```python
from build123d import *

# Parameters (mm, degrees)
SKETCH1_W           = 100
SKETCH1_H           = 100
SKETCH1_R           = 6
BOSS_EXTRUDE1_DEPTH = 4
SKETCH1_3_W         = 4
SKETCH1_3_H         = 99
SKETCH1_3_W_2       = 99
SKETCH1_3_H_2       = 4
BOSS_EXTRUDE3_DEPTH = 34
FILLET3_R           = 2
SKETCH2_R           = 2
SKETCH2_R_2         = 1.75
CUT_EXTRUDE1_DEPTH  = 4
SKETCH3_R           = 2
SKETCH3_R_2         = 1.75
CUT_EXTRUDE2_DEPTH  = 4
SKETCH4_R           = 2
SKETCH4_R_2         = 1.75
CUT_EXTRUDE3_DEPTH  = 4
SKETCH5_R           = 2
SKETCH5_R_2         = 1.75
CUT_EXTRUDE4_DEPTH  = 4


with BuildPart() as part:
    # Sketch1 → Boss-Extrude1 (new body)
    with BuildSketch(Plane.XY):
        with Locations((-48.16802168, -14.386178862)):
            Rectangle(SKETCH1_W, SKETCH1_H)
        with Locations((-88.16802168, -54.386178862)):
            Circle(SKETCH1_R, mode=Mode.SUBTRACT)
        with Locations((-8.16802168, -54.386178862)):
            Circle(SKETCH1_R, mode=Mode.SUBTRACT)
        with Locations((-8.16802168, 25.613821138)):
            Circle(SKETCH1_R, mode=Mode.SUBTRACT)
        with Locations((-88.16802168, 25.613821138)):
            Circle(SKETCH1_R, mode=Mode.SUBTRACT)
    extrude(amount=BOSS_EXTRUDE1_DEPTH)

    # Sketch1<3> → Boss-Extrude3 (add)
    with BuildSketch(Plane.XY):
        with Locations((-100.16802168, -14.386178862)):
            Rectangle(SKETCH1_3_W, SKETCH1_3_H)
        with Locations((-48.16802168, 37.613821138)):
            Rectangle(SKETCH1_3_W_2, SKETCH1_3_H_2)
        with Locations((3.83197832, -14.386178862)):
            Rectangle(SKETCH1_3_W, SKETCH1_3_H)
        with Locations((-48.16802168, -66.386178862)):
            Rectangle(SKETCH1_3_W_2, SKETCH1_3_H_2)
    extrude(amount=BOSS_EXTRUDE3_DEPTH)

    # Fillet3
    fillet3_edges = [part.edges().sort_by_distance(p)[0] for p in [
        (-102.16802168, -14.386178862, 0),
        (-48.16802168, 39.613821138, 0),
        (5.83197832, -14.386178862, 0),
        (-48.16802168, -68.386178862, 0),
    ]]
    fillet(fillet3_edges, radius=FILLET3_R)

    # Sketch2 → Cut-Extrude1 (cut)
    with BuildSketch(Plane.ZY.offset(102.16802168)):
        with Locations((25, 31.113821138)):
            Circle(SKETCH2_R)
        with Locations((25, -59.886178862)):
            Circle(SKETCH2_R)
        with Locations((11, 31.113821138)):
            Circle(SKETCH2_R)
        with Locations((11, -59.886178862)):
            Circle(SKETCH2_R)
        with Locations((11, 23.713821138)):
            Circle(SKETCH2_R_2)
        with Locations((11, -52.486178862)):
            Circle(SKETCH2_R_2)
    extrude(amount=-CUT_EXTRUDE1_DEPTH, mode=Mode.SUBTRACT)

    # Sketch3 → Cut-Extrude2 (cut)
    with BuildSketch(Plane.XZ.offset(68.386178862)):
        with Locations((-93.66802168, 25)):
            Circle(SKETCH3_R)
        with Locations((-2.66802168, 25)):
            Circle(SKETCH3_R)
        with Locations((-93.66802168, 11)):
            Circle(SKETCH3_R)
        with Locations((-2.66802168, 11)):
            Circle(SKETCH3_R)
        with Locations((-86.26802168, 11)):
            Circle(SKETCH3_R_2)
        with Locations((-9.56802168, 11)):
            Circle(SKETCH3_R_2)
    extrude(amount=-CUT_EXTRUDE2_DEPTH, mode=Mode.SUBTRACT)

    # Sketch4 → Cut-Extrude3 (cut)
    with BuildSketch(Plane(origin=(5.83197832, 0, 0), x_dir=(0, 0, -1), z_dir=(1, 0, 0))):
        with Locations((-25, -59.886178862)):
            Circle(SKETCH4_R)
        with Locations((-25, 31.113821138)):
            Circle(SKETCH4_R)
        with Locations((-11, -59.886178862)):
            Circle(SKETCH4_R)
        with Locations((-11, 31.113821138)):
            Circle(SKETCH4_R)
        with Locations((-11, -52.486178862)):
            Circle(SKETCH4_R_2)
        with Locations((-11, 23.713821138)):
            Circle(SKETCH4_R_2)
    extrude(amount=-CUT_EXTRUDE3_DEPTH, mode=Mode.SUBTRACT)

    # Sketch5 → Cut-Extrude4 (cut)
    with BuildSketch(Plane(origin=(0, 39.613821138, 0), x_dir=(1, 0, 0), z_dir=(0, 1, 0))):
        with Locations((-93.66802168, -25)):
            Circle(SKETCH5_R)
        with Locations((-2.66802168, -25)):
            Circle(SKETCH5_R)
        with Locations((-93.66802168, -11)):
            Circle(SKETCH5_R)
        with Locations((-2.66802168, -11)):
            Circle(SKETCH5_R)
        with Locations((-86.26802168, -11)):
            Circle(SKETCH5_R_2)
        with Locations((-10.06802168, -11)):
            Circle(SKETCH5_R_2)
    extrude(amount=-CUT_EXTRUDE4_DEPTH, mode=Mode.SUBTRACT)


solid = part.part
```
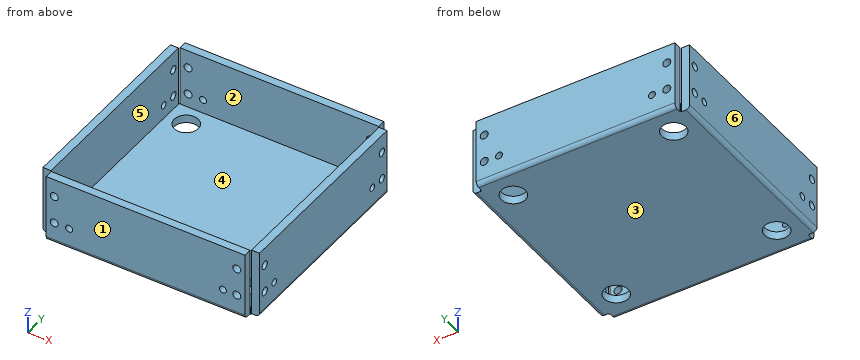
Read the model definition and answer for the solid it produces. Units are mm, in the model's axes. Face numbers are marked on the shaded views. A direction names the side the tool comes from. Round coordinates to 2 decimals unless told otherwise and drop trailing zeros. Write each loop counter-clockwise with the first axis right and the second up, starting at its lowest first coordinate (ties: lowest second). Pieces come first, ordered by that corner, then holes. Notation, with made-up numbers: (-9, -31.5) -> (49, -31.5) arc R33 cw to (49, 6.5) -> close; hole circle Ø10 at (51.5, -13.5). An arc over 180 degrees is marked (long way). Answer in a Markdown table with one row per item. Add a question column.
1) Find section C-C, the plane y = -6.5. Determine the outline of the cut face in (x, z).
2) Find section B-B, the plane x = -66.5. Determine the outline of the cut face in (y, z).
3) Find section D-D, the plane z = 25. State how many separate pieces and enclosed holes the cut face has, and give its area (3 significant figures).
4) Which of the six approach directions +Z, -Z, +X, -X, +Y, -Y give full straight-line access (tool end or side, diameter ignored) to the marked faces 1 and 2?
5) Given P1, Ø3, axis at y = -59.89, z = 11, coming from the -X side; P2, Ø4.5, axis at y = -66, z = 20, coming from the +X side, each flat-ended and moving along its own axis, determine where each tip first touches the part or whether it passes through.
6) Determine the mould class of the marked faces 3, 4, 5 and 6 for opening direction X: pulls with the +X half, pulls with the -X half, needs draft (parallel to the pull), parting line crosses it, or undercut.
7) Consider line 1 (Y direction, x = -100, z = 11); line 2 (Y direction, x = -31.5, z = 10.5); line 3 (X direction, y = -38.5, z = 19.5). Determine where each line is inside the solid, lowest interval first.
8) Find section A-A, the plane z = 6.5. Determine the outline of the cut face in (x, y).
Findings below:
| question | item | result |
|---|---|---|
| 1 | outline | (-102.17, 2) arc R2 ccw to (-100.17, 0) -> (3.83, 0) arc R2 ccw to (5.83, 2) -> (5.83, 34) -> (1.83, 34) -> (1.83, 4) -> (-98.17, 4) -> (-98.17, 34) -> (-102.17, 34) -> close |
| 2 | outline | (-68.39, 2) arc R2 ccw to (-66.39, 0) -> (37.61, 0) arc R2 ccw to (39.61, 2) -> (39.61, 34) -> (35.61, 34) -> (35.61, 4) -> (-64.39, 4) -> (-64.39, 34) -> (-68.39, 34) -> close |
| 3 | separate pieces | 12 |
| 3 | enclosed holes | 0 |
| 3 | area | 1,460 mm² |
| 4 | face 1 | +Z, -Z, +X, -X, -Y |
| 4 | face 2 | +Z, +X, -X |
| 5 | P1 | through |
| 5 | P2 | x = 5.83 |
| 6 | face 3 | needs draft |
| 6 | face 4 | undercut |
| 6 | face 5 | undercut |
| 6 | face 6 | pulls with the -X half |
| 7 | line 1 | -63.89 to -61.89, -57.89 to -54.24, -50.74 to 21.96, 25.46 to 29.11, 33.11 to 35.11 |
| 7 | line 2 | -68.39 to -64.39, 35.61 to 39.61 |
| 7 | line 3 | -102.17 to -98.17, 1.83 to 5.83 |
| 8 | outline | (-102.17, -63.89) -> (-98.17, -63.89) -> (-98.17, 35.11) -> (-102.17, 35.11) -> close; (-97.67, -68.39) -> (1.33, -68.39) -> (1.33, -64.39) -> (-97.67, -64.39) -> close; (-97.67, 35.61) -> (1.33, 35.61) -> (1.33, 39.61) -> (-97.67, 39.61) -> close; (1.83, -63.89) -> (5.83, -63.89) -> (5.83, 35.11) -> (1.83, 35.11) -> close |
